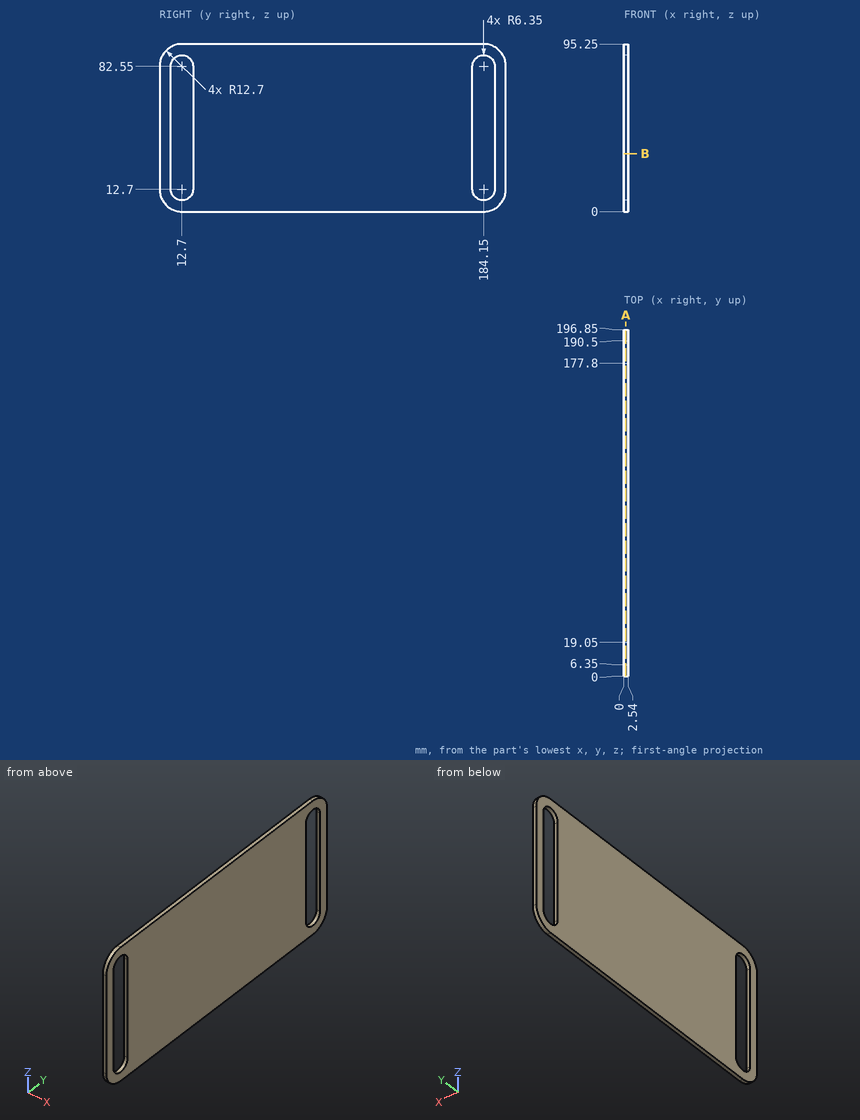
The drawing under review shows one solid part. Ordinate dimensions are in mm from its lowest x, y, z. Round coordinates to 2 decimals unless told otherwise and drop trailing zeros. Order: outer loops, then holes, each group sorted by start corner. A loop starts at its lowest first (then second) coordinate and runs counter-clockwise, first axis right, second up. Notation, with made-up numbers: (31, 63) -> (61, 63) arc R23 cw to (61, 87) -> close; hole circle Ø9 at (37.25, -21). An arc over 180 degrees is marked (long way). Return JSON: item names as keys, results as strings.
1. Take a section at A-A (x = 1.05). Write out the cut boundary in (y, z).
Answer block:
{"outline": "(0, 12.7) arc R12.7 ccw to (12.7, 0) -> (184.15, 0) arc R12.7 ccw to (196.85, 12.7) -> (196.85, 82.55) arc R12.7 ccw to (184.15, 95.25) -> (12.7, 95.25) arc R12.7 ccw to (0, 82.55) -> close; hole (6.35, 12.7) arc R6.35 ccw to (19.05, 12.7) -> (19.05, 82.55) arc R6.35 ccw to (6.35, 82.55) -> close; hole (177.8, 12.7) arc R6.35 ccw to (190.5, 12.7) -> (190.5, 82.55) arc R6.35 ccw to (177.8, 82.55) -> close"}
2. For L1, parallel to Y at x = 0.75, z = 28.5; L2, parallel to Y at x = 1.2, z = 8.5; L3, parallel to Z at x = 1.3, y = 13, list the stretches that pass through material, from the lowest coordinate up. Write a range as [from, to].
Answer block:
{"L1": "y = [0, 6.35], [19.05, 177.8], [190.5, 196.85]", "L2": "y = [0.71, 7.94], [17.46, 179.39], [188.91, 196.14]", "L3": "z = [0, 6.36], [88.89, 95.25]"}
3. Insertion check: P1, Ø4, axis at y = 141.5, z = 28, coming from the -X side. The pin has a flat end and moves straight along its axis. Give the tip position at first contact, or say it passes through.
Answer block:
{"P1": "stops at x = 0"}
4. Take a section at B-B (z = 33). Write out the cut boundary in (x, y).
Answer block:
{"outline": "(0, 0) -> (2.54, 0) -> (2.54, 6.35) -> (0, 6.35) -> close; (0, 19.05) -> (2.54, 19.05) -> (2.54, 177.8) -> (0, 177.8) -> close; (0, 190.5) -> (2.54, 190.5) -> (2.54, 196.85) -> (0, 196.85) -> close"}
